```python
from build123d import *

# Parameters (mm, degrees)
BOSS_EXTRUDE1_DEPTH      = 12
BOSS_EXTRUDE1_DEPTH_BACK = 10
CUT_EXTRUDE1_REACH       = 45.182
CUT_EXTRUDE1_START       = -2
SKETCH2_R                = 2.1


with BuildPart() as part:
    # Sketch1 → Boss-Extrude1 (new, two sides: drawn at the far end of the back side and taken through both)
    with BuildSketch(Plane.XY.offset(-BOSS_EXTRUDE1_DEPTH_BACK)):
        with BuildLine():
            Line((136.481143945, 38.574060338), (128.481143945, 38.574060338))
            Line((128.481143945, 38.574060338), (128.481143945, 18.574060338))
            Line((128.481143945, 18.574060338), (135.625186397, 18.574060338))
            add(Edge.make_bspline(
                [(136.481143945, 38.574060338), (136.479179267, 28.55738944), (135.625186397, 18.574060338)],
                knots=[0, 0, 0, 1, 1, 1], degree=2))
        make_face()
    extrude(amount=BOSS_EXTRUDE1_DEPTH + BOSS_EXTRUDE1_DEPTH_BACK)

    # Sketch2 → Cut-Extrude1 (cut, up to next)
    with BuildSketch(Plane.ZY.offset(-128.481143945).offset(CUT_EXTRUDE1_START), mode=Mode.PRIVATE) as cut_extrude1_sk1:
        with Locations((6, 28.574060338)):
            Circle(SKETCH2_R)
    cut_extrude1_tool1 = extrude(cut_extrude1_sk1.sketch, amount=-CUT_EXTRUDE1_REACH, mode=Mode.PRIVATE) & part.part
    add(cut_extrude1_tool1.solids().sort_by_distance((130.481144, 28.57406, 6))[0], mode=Mode.SUBTRACT)


solid = part.part
```
CAD build for the part. Positions are in the model's coordinates, mm. A direction names the side the tool comes from. Coordinates: 2 decimals unless noted, no trailing zeros. Order: outer loops, then holes, each group sorted by start corner. A loop starts at its lowest first (then second) coordinate and runs counter-clockwise, first axis right, second up. Notation, with made-up numbers: (52.25, 63.5) - (77.25, 63.5) arc R14 cw to (77.25, 85.5) - close; hole circle Ø1 at (30, 12.25). An arc over 180 degrees is marked (long way). Answer in a Markdown table with one row per item.
1. Drill centre lines: L1, parallel to X at y = 29, z = 5; L2, parallel to Y at x = 133.9, z = 6; L3, parallel to Z at x = 131.5, y = 27.5. Where is each one in solid material? Low to high. Write a range as from..to.
Answer:
| item | result |
|---|---|
| L1 | 128.48..130.48 |
| L2 | 18.57..26.47, 30.67..38.57 |
| L3 | -10..4.2, 7.8..12 |
2. Pull direction Y, two halves, no side cores. Call faces 1 (the face through (130.481, 29, 6)), 2 (the face through (133, 38.574, 1)), 3 (the face through (132, 29, 12)), 4 (the face through (132, 18.574, 1)): +Y half, -Y half, draft (parallel to the pull), parting line (faces both ways), or undercut.
Answer:
| item | result |
|---|---|
| face 1 | undercut |
| face 2 | +Y half |
| face 3 | draft |
| face 4 | -Y half |
3. 3-axis set-ups, long thin cutter, end or side, ignore diameter. For faces 5 (the face through (128.481, 29, 1)), 6 (the face through (133.373, 29.205, 8.003)): which of +Z, -Z, +X, -X, +Y, -Y reach the whole face in a straight line?
Answer:
| item | result |
|---|---|
| face 5 | +Z, -Z, -X, +Y, -Y |
| face 6 | +X |
4. Flat gauge pins, fed straight in: P1, Ø2, axis at y = 28.5, z = 7, coming from the +X side; P2, Ø12, axis at y = 27, z = 1.5, coming from the +X side; P3, Ø12, axis at y = 21.5, z = 7.5, coming from the +X side. Where does each tip first touch, or does it go through?
Answer:
| item | result |
|---|---|
| P1 | x = 130.48 |
| P2 | x = 136.41 |
| P3 | x = 136.22 |
5. Slice it at A-A, the plane x = 133.75. List the corners of the cut face in (y, z), then the cut area to 3 significant figures.
Answer:
| item | result |
|---|---|
| outline | (18.57, -10) - (38.57, -10) - (38.57, 12) - (18.57, 12) - close; hole circle Ø4.2 at (28.57, 6) |
| area | 426 mm² |
